from build123d import *

# Parameters (mm, degrees)
ESQUISSE1_W             = 235
ESQUISSE1_H             = 33
BOSS_EXTRU_1_DEPTH      = 10
ENL_V_MAT_EXTRU_1_DEPTH = 10


with BuildPart() as part:
    # Esquisse1 → Boss.-Extru.1 (new body)
    with BuildSketch(Plane.XY):
        Rectangle(ESQUISSE1_W, ESQUISSE1_H)
    extrude(amount=BOSS_EXTRU_1_DEPTH)

    # Esquisse2 → Enlèv. mat.-Extru.1 (cut)
    with BuildSketch(Plane.XY.offset(10)):
        Polygon((-117.5, 2), (-107.5, 2), (-107.5, 3.55), (-102, 3.55), (-102, 2), (-96, 2), (-96, -2), (-102, -2), (-102, -3.55), (-107.5, -3.55), (-107.5, -2), (-117.5, -2), align=None)
        Polygon((117.5, -2), (107.5, -2), (107.5, -3.55), (102, -3.55), (102, -2), (96, -2), (96, 2), (102, 2), (102, 3.55), (107.5, 3.55), (107.5, 2), (117.5, 2), align=None)
    extrude(amount=-ENL_V_MAT_EXTRU_1_DEPTH, mode=Mode.SUBTRACT)


solid = part.part
Model file for the job. Use its own axes, mm. A direction names the side the tool comes from. Round coordinates to 2 decimals unless told otherwise and drop trailing zeros. Loops run counter-clockwise (first coordinate to the right, second up) from the corner with the lowest first, then second, coordinate; pieces in that order, holes last. Notation, with made-up numbers: M 27.5,-7.5 L 33.5,-7.5 A18 ccw 33.5,-2.5 Z; hole C 37,18 d10. An arc over 180 degrees is marked long. One line per question, with ' | ' between items.
1) 3-axis set-ups, long thin cutter, end or side, ignore diameter. For faces 1 (the flat face through (-113, 2, 5)), 2 (the flat face through (99, 2, 5)), 3 (the flat face through (-105, -3.55, 5)): which of +Z, -Z, +X, -X, +Y, -Y reach the whole face in a straight line?
Solved:
face 1: +Z, -Z, -X | face 2: +Z, -Z, +X | face 3: +Z, -Z
2) Band-saw the part on A-A (z = 8.5). Give the cut face in (x, y), then the cut area to 3 significant figures.
Solved:
outline: M -117.5,-16.5 L 117.5,-16.5 L 117.5,-2 L 107.5,-2 L 107.5,-3.55 L 102,-3.55 L 102,-2 L 96,-2 L 96,2 L 102,2 L 102,3.55 L 107.5,3.55 L 107.5,2 L 117.5,2 L 117.5,16.5 L -117.5,16.5 L -117.5,2 L -107.5,2 L -107.5,3.55 L -102,3.55 L -102,2 L -96,2 L -96,-2 L -102,-2 L -102,-3.55 L -107.5,-3.55 L -107.5,-2 L -117.5,-2 Z | area: 7,550 mm²
3) Drill centre lines: line 1 along X through (y, z) = (2.5, 7.75); line 2 along Y through (x, z) = (-104, 5.5). Where is each one in solid material? Low to high.
Solved:
line 1: x = -117.5 to -107.5, -102 to 102, 107.5 to 117.5 | line 2: y = -16.5 to -3.55, 3.55 to 16.5
4) Flat gauge pin, fed straight in: pin 1 (1 mm diameter, centred on x = 25, y = -7.5, fed in from -Z). Where does the tip first touch, or does it go through?
Solved:
pin 1: stops at z = 0
5) Mould opens along Y. For faces 4 (the flat face through (96, 0, 5)), 5 (the flat face through (117.5, -9, 5)), 6 (the flat face through (-2, 16.5, 5)) say: +Y half, -Y half, draft (parallel to the pull), parting line (faces both ways), or undercut.
Solved:
face 4: undercut | face 5: draft | face 6: +Y half
6) Band-saw the part on B-B (y = 0). Give the cut face in (x, z), then the cut area to 3 significant figures.
Solved:
outline: M -96,0 L 96,0 L 96,10 L -96,10 Z | area: 1,920 mm²
